Source: CAD feature listing. Evaluate the final solid. Frame: model axes, mm. Give positions to 0.01 mm unless a question says otherwise; leave off trailing zeros. Write each loop counter-clockwise with the first axis right and the second up, starting at its lowest first coordinate (ties: lowest second). Pieces come first, ordered by that corner, then holes. Notation, with made-up numbers: (32.5, 80) -> (69.5, 80) arc R18 ccw to (69.5, 100) -> close; hole circle Ø8 at (-16, 60). An arc over 180 degrees is marked (long way). Write item = value, one per line.
from build123d import *

# Parameters (mm, degrees)
SKETCH_1_R             = 5
EXTRUDE_1_DEPTH        = 2
SHELL_1_T              = -1
FILLET_1_R             = 0.5
FILLET_2_R             = 1
HOLE_WIZARD_M2_1_D     = 1.6
HOLE_WIZARD_M2_1_DEPTH = 5.2
HOLE_WIZARD_M2_1_TIP   = 0.480688495


with BuildPart() as part:
    # 草图1 → 凸台-拉伸1 (new body)
    with BuildSketch(Plane.XY):
        Circle(SKETCH_1_R)
    extrude(amount=EXTRUDE_1_DEPTH)

    # 抽壳1
    shell_1_openings = [part.faces().sort_by_distance(p)[0] for p in [
        (0, 0, 2),
    ]]
    offset(amount=SHELL_1_T, openings=shell_1_openings, kind=Kind.INTERSECTION)

    # 圆角1
    fillet_1_edges = [part.edges().sort_by_distance(p)[0] for p in [
        (-4, 0, 1),
    ]]
    fillet(fillet_1_edges, radius=FILLET_1_R)

    # 圆角2
    fillet_2_edges = [part.edges().sort_by_distance(p)[0] for p in [
        (-5, 0, 0),
    ]]
    fillet(fillet_2_edges, radius=FILLET_2_R)

    # M2 螺纹孔1
    with Locations(Plane.XY.offset(1)):
        with Locations((0, 0)):
            Hole(HOLE_WIZARD_M2_1_D / 2, depth=HOLE_WIZARD_M2_1_DEPTH)
            with Locations((0, 0, -(HOLE_WIZARD_M2_1_DEPTH + HOLE_WIZARD_M2_1_TIP / 2))):  # 118° drill point
                Cone(0, HOLE_WIZARD_M2_1_D / 2, HOLE_WIZARD_M2_1_TIP, mode=Mode.SUBTRACT)


solid = part.part
1) Material intervals for L1, parallel to Y at x = 0, z = 1.7; L2, parallel to Z at x = 1.5, y = 2.5; L3, parallel to X at y = 0.75, z = 1.95, sorted ascending.
Computed:
L1 = -5 to -4, 4 to 5
L2 = 0 to 1
L3 = -4.94 to -3.93, 3.93 to 4.94
2) Draft query along X for faces 1 (the cylindrical face through (-1.08, -4.88, 1.49)), 2 (the flat face through (0, 1, 1)), 3 (the flat face through (1, 0, 0)), 4 (the cylindrical face through (-0.867, -3.905, 1.746)). Return one class per face: pulls with the +X half, pulls with the -X half, needs draft (parallel to the pull), parting line crosses it, or undercut.
Computed:
face_1 = parting line crosses it
face_2 = undercut
face_3 = needs draft
face_4 = undercut
3) Cut plane A-A (y = 0). Return the cut outline in (x, z).
Computed:
outline = (-5, 1) arc R1 ccw to (-4, 0) -> (-0.8, 0) -> (-0.8, 1) -> (-3.5, 1) arc R0.5 cw to (-4, 1.5) -> (-4, 2) -> (-5, 2) -> close; (0.8, 0) -> (4, 0) arc R1 ccw to (5, 1) -> (5, 2) -> (4, 2) -> (4, 1.5) arc R0.5 cw to (3.5, 1) -> (0.8, 1) -> close
4) Cut plane D-D (z = 0.6). Return the cut outline in (x, y).
Computed:
outline = circle Ø9.83 at (0, 0); hole circle Ø1.6 at (0, 0)
5) Cut plane C-C (z = 1.15). Return the cut outline in (x, y).
Computed:
outline = circle Ø10 at (0, 0); hole circle Ø7.71 at (0, 0)
6) Contact query for flat-ended pins moving along their axis: pin 1 (1 mm diameter, centred on x = 0, y = 0, fed in from +Z); pin 2 (1.5 mm diameter, centred on x = 1, y = 0, fed in from +Z). Output: stop coordinate, or through.
Computed:
pin_1 = through
pin_2 = 1
